Source: CAD feature listing. Evaluate the final solid. Frame: model axes, mm. Face numbers are marked on the shaded views. Give positions to 0.01 mm unless a question says otherwise; leave off trailing zeros. Order: outer loops, then holes, each group sorted by start corner. A loop starts at its lowest first (then second) coordinate and runs counter-clockwise, first axis right, second up. Notation, with made-up numbers: (-4, 40.25) -> (26, 40.25) arc R15 ccw to (26, 59.25) -> close; hole circle Ø5 at (-28, -27.5). An arc over 180 degrees is marked (long way). Answer in a Markdown table with one row per item.
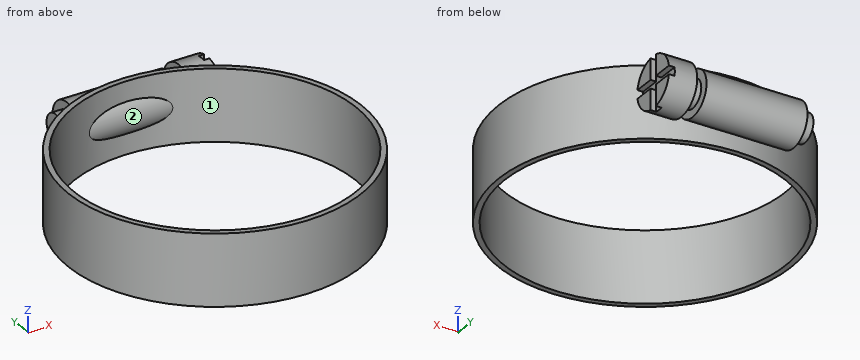
```python
from build123d import *

# Parameters (mm, degrees)
SKETCH1_W                = 12.7
SKETCH1_H                = 1
SKETCH2_R                = 4
BOSS_EXTRUDE1_DEPTH      = 9
BOSS_EXTRUDE2_DEPTH      = 2
BOSS_EXTRUDE2_DEPTH_BACK = 20
SKETCH3_R                = 2.5
SKETCH4_R                = 4.540800692
BOSS_EXTRUDE3_DEPTH      = 5
CUT_EXTRUDE1_DEPTH       = 1


with BuildPart() as part:
    # Sketch1 → Revolve1 (revolve)
    with BuildSketch(Plane(origin=(0, 0, 0), x_dir=(0, 0, -1), z_dir=(1, 0, 0)), mode=Mode.PRIVATE) as revolve1_sk:
        with Locations((0, 25.5)):
            Rectangle(SKETCH1_W, SKETCH1_H)
    revolve(revolve1_sk.sketch.rotate(Axis((0, 0, 0), (0, 0, -1)), 90), axis=Axis((0, 0, 0), (0, 0, -1)))

    # Sketch2 → Boss-Extrude1 (add, symmetric)
    with BuildSketch(Plane(origin=(0, 0, 0), x_dir=(0, 0, -1), z_dir=(1, 0, 0))):
        with Locations((0, 27.867620805)):
            Circle(SKETCH2_R)
    extrude(amount=BOSS_EXTRUDE1_DEPTH, both=True)

    # Sketch3 → Boss-Extrude2 (add, two sides: drawn at the far end of the back side and taken through both)
    with BuildSketch(Plane(origin=(9, 0, 0), x_dir=(0, 0, -1), z_dir=(1, 0, 0)).offset(-BOSS_EXTRUDE2_DEPTH_BACK)):
        with Locations((0, 27.867620805)):
            Circle(SKETCH3_R)
    extrude(amount=BOSS_EXTRUDE2_DEPTH + BOSS_EXTRUDE2_DEPTH_BACK)

    # Sketch4 → Boss-Extrude3 (add)
    with BuildSketch(Plane(origin=(11, 0, 0), x_dir=(0, 0, -1), z_dir=(1, 0, 0))):
        with Locations(Location((0, 27.867620805, 0), (0, 0, 251.621037372))):
            Circle(SKETCH4_R)
    extrude(amount=BOSS_EXTRUDE3_DEPTH)

    # Sketch5 → Cut-Extrude1 (cut)
    with BuildSketch(Plane(origin=(16, 0, 0), x_dir=(0, 0, -1), z_dir=(1, 0, 0))):
        Polygon((0.75, 27.117620805), (5.588794468, 27.117620805), (5.588794468, 28.617620805), (0.75, 28.617620805), (0.75, 32.881878849), (-0.75, 32.881878849), (-0.75, 28.617620805), (-5.588794468, 28.617620805), (-5.588794468, 27.117620805), (-0.75, 27.117620805), (-0.75, 22.853362761), (0.75, 22.853362761), align=None)
    extrude(amount=-CUT_EXTRUDE1_DEPTH, mode=Mode.SUBTRACT)


solid = part.part
```
(1) First-contact query: pin 1 Ø1.5 at (x, z) = (-0.5, 5) entering from -Y; pin 2 Ø7.5 at (y, z) = (29.5, -1.5) entering from +X; pin 3 Ø2 at (y, z) = (27.5, 1.5) entering from -X. Flat tips, straight axial feed; report the tip coordinate or a pass-through.
A:
| item | result |
|---|---|
| pin 1 | stops at y = -26 |
| pin 2 | stops at x = 16 |
| pin 3 | stops at x = -11 |
(2) Section query B-B (x = -3.5). Return the cut outline in (y, z).
A:
| item | result |
|---|---|
| outline | (-25.76, -6.35) -> (-24.75, -6.35) -> (-24.75, 6.35) -> (-25.76, 6.35) -> close; (24.75, -6.35) -> (25.76, -6.35) -> (25.76, -3.4) arc R4 ccw (long way) to (25.76, 3.4) -> (25.76, 6.35) -> (24.75, 6.35) -> (24.75, 2.51) arc R4 ccw to (24.75, -2.51) -> close |
(3) Section query C-C (z = 0). Return the cut outline in (x, y), plus the area to 3 significant figures.
A:
| item | result |
|---|---|
| outline | (-11, 25.37) -> (-9, 25.37) -> (-9, 24.39) arc R26 ccw (long way) to (11.48, 23.33) -> (15, 23.33) -> (15, 32.41) -> (11, 32.41) -> (11, 30.37) -> (9, 30.37) -> (9, 31.87) -> (-9, 31.87) -> (-9, 30.37) -> (-11, 30.37) -> close; hole (-7.44, 23.87) arc R25 ccw (long way) to (7.44, 23.87) -> close; hole (9, 24.39) arc R26 cw to (11, 23.56) -> (11, 25.37) -> (9, 25.37) -> close |
| area | 343 mm^2 |
(4) Section query D-D (x = 14). Return the cut outline in (y, z), plus the area to 3 significant figures.
A:
| item | result |
|---|---|
| outline | (-21.91, -6.35) -> (-20.71, -6.35) -> (-20.71, 6.35) -> (-21.91, 6.35) -> close; (20.71, -6.35) -> (21.91, -6.35) -> (21.91, 6.35) -> (20.71, 6.35) -> close; circle Ø9.08 at (27.87, 0) |
| area | 95.2 mm^2 |
(5) Section query A-A (y = 0). Return the cut outline in (x, z).
A:
| item | result |
|---|---|
| outline | (-26, -6.35) -> (-25, -6.35) -> (-25, 6.35) -> (-26, 6.35) -> close; (25, -6.35) -> (26, -6.35) -> (26, 6.35) -> (25, 6.35) -> close |
(6) Pull-direction query (X, two-part tool) for the marked faces 1 and 2; classes: +X half, -X half, draft (parallel to the pull), parting line (faces both ways), or undercut.
A:
| item | result |
|---|---|
| face 1 | undercut |
| face 2 | undercut |
(7) Ray query, probe 1 along Y at (x, z) = (11.5, -3); probe 2 along X at (y, z) = (-15, 1); probe 3 along X at (y, z) = (11, 1.5). Return the intervals inside material, ascending.
A:
| item | result |
|---|---|
| probe 1 | y = -23.32 to -22.2, 22.2 to 23.32, 24.46 to 31.28 |
| probe 2 | x = -21.24 to -20, 20 to 21.24 |
| probe 3 | x = -23.56 to -22.45, 22.45 to 23.56 |
